```python
from build123d import *

# Parameters (mm, degrees)
ESQUISSE1_R                         = 5
ESQUISSE1_R_2                       = 2.5
BOSS_EXTRU_1_DEPTH                  = 20
ESQUISSE2_R                         = 2.5
BOSS_EXTRU_2_DEPTH                  = 70
BOSS_EXTRU_2_DIRECTION_2_REACH      = 24.913
BOSS_EXTRU_2_DIRECTION_2_END_RADIUS = 5


with BuildPart() as part:
    # Esquisse1 → Boss.-Extru.1 (new body)
    with BuildSketch(Plane.XY):
        Circle(ESQUISSE1_R)
        Circle(ESQUISSE1_R_2, mode=Mode.SUBTRACT)
    extrude(amount=BOSS_EXTRU_1_DEPTH)

    # Esquisse2 → Boss.-Extru.2 (add)
    with BuildSketch(Plane(origin=(5, 0, 0), x_dir=(0, 0, -1), z_dir=(1, 0, 0))):
        with Locations((-10, 0)):
            Circle(ESQUISSE2_R)
    extrude(amount=BOSS_EXTRU_2_DEPTH)

    # Boss.-Extru.2 direction 2: up to this cylinder (the profile starts outside it)
    boss_extru_2_direction_2_end = Plane(origin=(0, 0, 10), z_dir=(0, 0, -1)) * Cylinder(BOSS_EXTRU_2_DIRECTION_2_END_RADIUS, 60.826, mode=Mode.PRIVATE)
    # Esquisse2 → Boss.-Extru.2 direction 2 (add, up to the surface)
    with BuildSketch(Plane(origin=(5, 0, 0), x_dir=(0, 0, -1), z_dir=(1, 0, 0)), mode=Mode.PRIVATE) as boss_extru_2_direction_2_sk1:
        with Locations((-10, 0)):
            Circle(ESQUISSE2_R)
    boss_extru_2_direction_2_tool1 = extrude(boss_extru_2_direction_2_sk1.sketch, amount=-BOSS_EXTRU_2_DIRECTION_2_REACH, mode=Mode.PRIVATE) - boss_extru_2_direction_2_end
    add(boss_extru_2_direction_2_tool1.solids().sort_by_distance((5, 0, 10))[0])
    add(boss_extru_2_direction_2_tool1.solids().sort_by_distance((5, 0, 10))[1])


solid = part.part
```
Verification items for the finished model (mm, model axes). Round coordinates to 2 decimals unless told otherwise and drop trailing zeros. Write each loop counter-clockwise with the first axis right and the second up, starting at its lowest first coordinate (ties: lowest second). Pieces come first, ordered by that corner, then holes.
1. Section check B-B on z = 10. Enter the section's corners in (x, y).
2. Draft check along X on faces 1 (the cylindrical face through (-5, 0, 10)), 2 (the cylindrical face through (-0.54, -2.44, 9.86)), 3 (the flat face through (75, 0, 10)). Enter one of: +X half, -X half, draft (parallel to the pull), parting line (faces both ways), or undercut.
3. Section check D-D on x = 15. Enter the section's corners in (y, z), plus the area to 3 significant figures.
4. Gauge pin test, flat ends, axial feed: P1, Ø4, axis at x = 13, z = 4, coming from the -Y side; P2, Ø1.5, axis at y = 4, z = 13.5, coming from the -X side; P3, Ø3, axis at x = 38.5, y = 1, coming from the -Z side; P4, Ø2, axis at x = 46, y = 2, coming from the +Z side. Record the tip position at first contact, or that the pin passes through.
5. Scan lines: L1, parallel to Y at x = 0, z = 11.75; L2, parallel to X at y = 2.25, z = 11; L3, parallel to X at y = 1.5, z = 5. Record each from-to range of solid material in increasing order.
6. Section check C-C on y = 1.75. Enter the section's corners in (x, z), plus the area to 3 significant figures.
7. Section check A-A on x = 0. Enter the section's corners in (y, z), plus the area to 3 significant figures.
Answer:
1. outline: (4.33, -2.5) - (75, -2.5) - (75, 2.5) - (4.33, 2.5) arc R5 ccw (long way) to start; hole circle Ø5 at (0, 0)
2. face 1: parting line
2. face 2: undercut
2. face 3: +X half
3. outline: circle Ø5 at (0, 10)
3. area: 19.6 mm2
4. P1: passes through
4. P2: stops at x = -3.8
4. P3: stops at z = 7.5
4. P4: stops at z = 12.29
5. L1: y = -5 to -2.5, 2.5 to 5
5. L2: x = -4.47 to -1.09, 1.09 to 75
5. L3: x = -4.77 to -2, 2 to 4.77
6. outline: (-4.68, 0) - (-1.79, 0) - (-1.79, 20) - (-4.68, 20) - close; (1.79, 0) - (4.68, 0) - (4.68, 8.21) - (75, 8.21) - (75, 11.79) - (4.68, 11.79) - (4.68, 20) - (1.79, 20) - close
6. area: 367 mm2
7. outline: (-5, 0) - (-2.5, 0) - (-2.5, 20) - (-5, 20) - close; (2.5, 0) - (5, 0) - (5, 20) - (2.5, 20) - close
7. area: 100 mm2
